```python
from build123d import *

# Parameters (mm, degrees)
BOSS_EXTRUDE1_DEPTH             = 5.08
F_1_4_0_25_DIAMETER_HOLE1_D     = 6.35
F_1_4_0_25_DIAMETER_HOLE1_DEPTH = 25.4
F_1_4_0_25_DIAMETER_HOLE1_TIP   = 1.907732465
CUT_EXTRUDE1_DEPTH              = 108.882743755
CUT_EXTRUDE1_DEPTH_BACK         = 108.882743755
SKETCH5_W                       = 25.4
SKETCH5_H                       = 5.08


with BuildPart() as part:
    # Sketch1 → Boss-Extrude1 (new body)
    with BuildSketch(Plane(origin=(0, 0, 0), x_dir=(1, 0, 0), z_dir=(0, 1, 0))):
        Polygon((0, 0), (0, 76.2), (25.4, 76.2), (25.4, 25.4), (76.2, 25.4), (76.2, 0), align=None)
    extrude(amount=BOSS_EXTRUDE1_DEPTH)

    # 1/4 (0.25) Diameter Hole1
    with Locations(Plane(origin=(0, 5.08, 0), x_dir=(1, 0, 0), z_dir=(0, 1, 0))):
        with Locations((12.7, 63.5), (12.7, 38.1), (12.7, 12.7), (38.1, 12.7), (63.5, 12.7)):
            Hole(F_1_4_0_25_DIAMETER_HOLE1_D / 2, depth=F_1_4_0_25_DIAMETER_HOLE1_DEPTH)
            with Locations((0, 0, -(F_1_4_0_25_DIAMETER_HOLE1_DEPTH + F_1_4_0_25_DIAMETER_HOLE1_TIP / 2))):  # 118° drill point
                Cone(0, F_1_4_0_25_DIAMETER_HOLE1_D / 2, F_1_4_0_25_DIAMETER_HOLE1_TIP, mode=Mode.SUBTRACT)

    # Sketch5 → Cut-Extrude1 (cut, two sides: drawn at the far end of the back side and taken through both)
    with BuildSketch(Plane(origin=(0, 0, -76.2), x_dir=(-1, 0, 0), z_dir=(0, 0, -1)).offset(-CUT_EXTRUDE1_DEPTH_BACK)):
        with Locations((-12.7, 2.54)):
            Rectangle(SKETCH5_W, SKETCH5_H)
    extrude(amount=CUT_EXTRUDE1_DEPTH + CUT_EXTRUDE1_DEPTH_BACK, mode=Mode.SUBTRACT)


solid = part.part
```
Could you check a few things on this model? Use its own coordinates, in mm. Round coordinates to 2 decimals unless told otherwise and drop trailing zeros. Loops run counter-clockwise (first coordinate to the right, second up) from the corner with the lowest first, then second, coordinate; pieces in that order, holes last.
Q1. I want a section at D-D (z = -15.25). Write out the boundary of the cut face in (x, y), and give its area (3 significant figures).
Q2. I want a section at C-C (y = 3.25). Write out the boundary of the cut face in (x, z) (3 decimals), and give its area (3 significant figures).
Q3. Please list where these lines run through material, in increasing order: L1, parallel to X at y = 2.35, z = -12.7 (3 decimals); L2, parallel to Z at x = 63.5, y = 2.8 (3 decimals); L3, parallel to X at y = 1.25, z = -14.5.
Q4. I want a section at A-A (x = 38.1). Write out the boundary of the cut face in (y, z) (3 decimals), and give its area (3 significant figures).
Q5. I want a section at B-B (z = -12.7). Write out the boundary of the cut face in (x, y) (3 decimals), and give its area (3 significant figures).
Q6. Thinking about a two-plate mould opening in X: for faces 1 (the flat face through (76.2, 3, -13)), 2 (the cylindrical face through (60.57, 2.5, -11.48)), 3 (the flat face through (50, 3, -25.4)), which applies, pulls with the +X half, pulls with the -X half, needs draft (parallel to the pull), parting line crosses it, or undercut?
Q7. For P1, Ø5, axis at x = 63.5, z = -12.7, coming from the -Y side, with a flat end and sliding along its axis, tell me the tip position at first contact or that it passes through.
Answer below:
1. outline: (25.4, 0) - (36.21, 0) - (36.21, 5.08) - (25.4, 5.08) - close; (39.99, 0) - (61.61, 0) - (61.61, 5.08) - (39.99, 5.08) - close; (65.39, 0) - (76.2, 0) - (76.2, 5.08) - (65.39, 5.08) - close
1. area: 220 mm2
2. outline: (25.4, -25.4) - (76.2, -25.4) - (76.2, 0) - (25.4, 0) - close; hole circle Ø6.35 at (38.1, -12.7); hole circle Ø6.35 at (63.5, -12.7)
2. area: 1,230 mm2
3. L1: x = 25.4 to 34.925, 41.275 to 60.325, 66.675 to 76.2
3. L2: z = -25.4 to -15.875, -9.525 to 0
3. L3: x = 25.4 to 35.48, 40.72 to 60.88, 66.12 to 76.2
4. outline: (0, -25.4) - (5.08, -25.4) - (5.08, -15.875) - (0, -15.875) - close; (0, -9.525) - (5.08, -9.525) - (5.08, 0) - (0, 0) - close
4. area: 96.8 mm2
5. outline: (25.4, 0) - (34.925, 0) - (34.925, 5.08) - (25.4, 5.08) - close; (41.275, 0) - (60.325, 0) - (60.325, 5.08) - (41.275, 5.08) - close; (66.675, 0) - (76.2, 0) - (76.2, 5.08) - (66.675, 5.08) - close
5. area: 194 mm2
6. face 1: pulls with the +X half
6. face 2: undercut
6. face 3: needs draft
7. P1: passes through
